Design review of the part built by this model. Coordinates are the model's own, in mm. Face numbers are marked on the shaded views. A direction names the side the tool comes from. Round coordinates to 2 decimals unless told otherwise and drop trailing zeros. Order: outer loops, then holes, each group sorted by start corner. A loop starts at its lowest first (then second) coordinate and runs counter-clockwise, first axis right, second up.
from build123d import *

# Parameters (mm, degrees)
BOX038_W               = 4.1
BOX038_H               = 5
BOX038_DEPTH           = 2
BOX038_PLACEMENT_ANGLE = 20
BOX037_W               = 2.85
BOX037_H               = 2.4
BOX037_DEPTH           = 1.5
BOX036_W               = 12
BOX036_H               = 1
BOX036_DEPTH           = 5
SKETCH035_W            = 3
SKETCH035_H            = 1.2
EXTRUDE005_DEPTH       = 10.8
BOX007_W               = 15.8
BOX007_H               = 20.8
BOX007_DEPTH           = 13.2
FILLET008_R            = 0.1


with BuildPart() as cube017:
    # Box038 → Box038 (new body)
    with BuildSketch(Plane.XY):
        with Locations((2.05, 2.5)):
            Rectangle(BOX038_W, BOX038_H)
    extrude(amount=BOX038_DEPTH)


with BuildPart() as cube017_1:
    # Box038 placement: moved
    add(cube017.part.moved(Location((-2.05, -1, 11.2))).rotate(Axis((-2.05, -1, 11.2), (-1, 0, 0)), BOX038_PLACEMENT_ANGLE))


with BuildPart() as cube016:
    # Box037 → Box037 (new body)
    with BuildSketch(Plane(origin=(3.15, 8.4, 8.2), x_dir=(1, 0, 0), z_dir=(0, 0, 1))):
        with Locations((1.425, 1.2)):
            Rectangle(BOX037_W, BOX037_H)
    extrude(amount=BOX037_DEPTH)


with BuildPart() as cube041:
    # Clone base: copy of Cube016
    add(cube016.part)


with BuildPart() as cube041_1:
    # Clone placement: moved
    add(cube041.part.moved(Location((-9.15, 0, 0))))


with BuildPart() as fusion024:
    # Box036 → Box036 (new body)
    with BuildSketch(Plane(origin=(-6, 9.8, 2.7), x_dir=(1, 0, 0), z_dir=(0, 0, 1))):
        with Locations((6, 0.5)):
            Rectangle(BOX036_W, BOX036_H)
    extrude(amount=BOX036_DEPTH)

    # Fusion024: union Cube016, Cube041
    add(cube016.part)
    add(cube041_1.part)


with BuildPart() as fusion025:
    # Sketch035 → Extrude005 (new body)
    with BuildSketch(Plane.XZ):
        Polygon((-6, 9.7), (-6, 2.7), (6, 2.7), (6, 9.7), (3.15, 9.7), (3.15, 11.3), (2.05, 11.3), (2.05, 12.5), (-2.05, 12.5), (-2.05, 11.3), (-3.15, 11.3), (-3.15, 9.7), align=None)
        with Locations((-5.3, 11.1)):
            Rectangle(SKETCH035_W, SKETCH035_H)
        with Locations((5.3, 11.1)):
            Rectangle(SKETCH035_W, SKETCH035_H)
    extrude(amount=-EXTRUDE005_DEPTH)

    # Cut001: cut Fusion024
    add(fusion024.part, mode=Mode.SUBTRACT)

    # Fusion025: union Cube017
    add(cube017_1.part)


with BuildPart() as fusion025_1:
    # Fusion025 placement: moved
    add(fusion025.part.moved(Location((0, 0.1, 0.1))))


with BuildPart() as body009:
    # Box007 → Box007 (new body)
    with BuildSketch(Plane(origin=(-7.9, 0.2, 0.2), x_dir=(1, 0, 0), z_dir=(0, 0, 1))):
        with Locations((7.9, 10.4)):
            Rectangle(BOX007_W, BOX007_H)
    extrude(amount=BOX007_DEPTH)

    # Fillet008
    fillet008_edges = [body009.edges().sort_by_distance(p)[0] for p in [
        (-7.9, 0.2, 6.8),
        (-7.9, 21, 6.8),
        (-7.9, 10.6, 0.2),
        (7.9, 0.2, 6.8),
        (7.9, 21, 6.8),
        (7.9, 10.6, 0.2),
        (0, 0.2, 0.2),
        (0, 21, 0.2),
    ]]
    fillet(fillet008_edges, radius=FILLET008_R)

    # Cut008: cut Fusion025
    add(fusion025_1.part, mode=Mode.SUBTRACT)


solid = body009.part
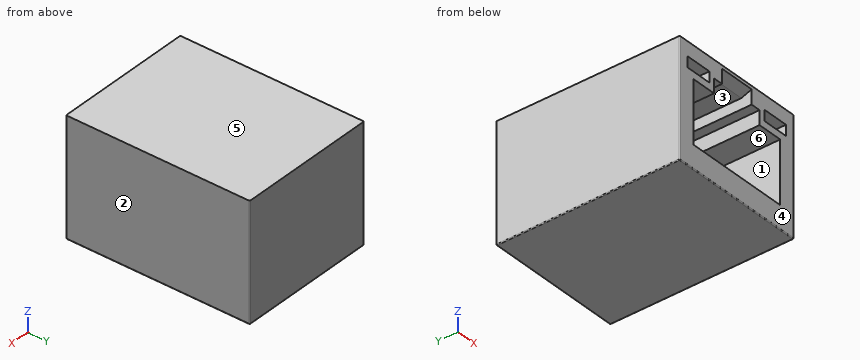
1) Take a section at C-C on x = -2.5. Give the boundary of the cut face in (y, z), plus the area to 3 significant figures.
Results:
outline: (0.2, 0.3) arc R0.1 ccw to (0.3, 0.2) - (20.9, 0.2) arc R0.1 ccw to (21, 0.3) - (21, 13.4) - (0.2, 13.4) - (0.2, 11.4) - (10.9, 11.4) - (10.9, 7.8) - (9.9, 7.8) - (9.9, 2.8) - (0.2, 2.8) - close
area: 188 mm2
2) The part is to be moulded in two halves that separate along Z. For the marked faces 3, 4, 5 and 6, say which applies: released by +Z, released by -Z, zero draft, split by the parting line, or undercut.
Results:
face 3: undercut
face 4: zero draft
face 5: released by +Z
face 6: undercut
3) To check wall thickness, follow line 1 along Z through (x, y) = (-4, 7); line 2 along X through (y, z) = (8, 9); line 3 along X through (y, z) = (5.5, 10). State the ranges of each line that lie inside material, in increasing order.
Results:
line 1: z = 0.2 to 2.8, 9.8 to 10.6, 11.8 to 13.4
line 2: x = -7.9 to -6, 6 to 7.9
line 3: x = -7.9 to -3.15, 3.15 to 7.9
4) Take a section at A-A on y = 2.5. Give the boundary of the cut face in (x, z), plus the area to 3 significant figures.
Results:
outline: (-7.9, 0.3) arc R0.1 ccw to (-7.8, 0.2) - (7.8, 0.2) arc R0.1 ccw to (7.9, 0.3) - (7.9, 13.4) - (-7.9, 13.4) - close; hole (-6.8, 10.6) - (-3.8, 10.6) - (-3.8, 11.8) - (-6.8, 11.8) - close; hole (-6, 2.8) - (6, 2.8) - (6, 9.8) - (3.15, 9.8) - (3.15, 11.4) - (2.05, 11.4) - (2.05, 12.6) - (-2.05, 12.6) - (-2.05, 11.4) - (-3.15, 11.4) - (-3.15, 9.8) - (-6, 9.8) - close; hole (3.8, 10.6) - (6.8, 10.6) - (6.8, 11.8) - (3.8, 11.8) - close
area: 102 mm2
5) Clearance check with flat-ended pins moving along their axes: P1, Ø5.5, axis at x = -2, z = 4, coming from the -Y side; P2, Ø2, axis at x = -4, z = 6.5, coming from the -Y side. State where each tip first meets the part, or that it passes through.
Results:
P1: stops at y = 0.2
P2: stops at y = 9.9
6) Take a section at B-B on z = 12.25. Give the boundary of the cut face in (x, y).
Results:
outline: (-7.9, 0.3) arc R0.1 ccw to (-7.8, 0.2) - (-2.05, 0.2) - (-2.05, 10.9) - (2.05, 10.9) - (2.05, 0.2) - (7.8, 0.2) arc R0.1 ccw to (7.9, 0.3) - (7.9, 20.9) arc R0.1 ccw to (7.8, 21) - (-7.8, 21) arc R0.1 ccw to (-7.9, 20.9) - close
7) Take a section at D-D on x = -5.75. Give the boundary of the cut face in (y, z).
Results:
outline: (0.2, 0.3) arc R0.1 ccw to (0.3, 0.2) - (20.9, 0.2) arc R0.1 ccw to (21, 0.3) - (21, 13.4) - (0.2, 13.4) - (0.2, 11.8) - (10.9, 11.8) - (10.9, 10.6) - (0.2, 10.6) - (0.2, 9.8) - (8.5, 9.8) - (8.5, 8.3) - (10.9, 8.3) - (10.9, 7.8) - (9.9, 7.8) - (9.9, 2.8) - (0.2, 2.8) - close
8) For the marked faces 1 and 2, list the 3-axis set-ups (+Z, -Z, +X, -X, +Y, -Y) from which the entire face can be reached by the end or side of a thin tool; tool diameter is ignored.
Results:
face 1: -Y
face 2: +Z, -Z, +X, +Y, -Y
